Read the model definition and answer for the solid it produces. Units are mm, in the model's axes. A direction names the side the tool comes from. Round coordinates to 2 decimals unless told otherwise and drop trailing zeros. Write each loop counter-clockwise with the first axis right and the second up, starting at its lowest first coordinate (ties: lowest second). Pieces come first, ordered by that corner, then holes. Notation, with made-up numbers: (83.25, -30.5) - (117.25, -30.5) arc R5 ccw to (117.25, -22.5) - close; hole circle Ø6 at (31, 60.5). An arc over 180 degrees is marked (long way). One line per item, written item: value. Start each with the question number.
(1) A cutting plane is placed at C-C, the plane y = 11. Determine the outline of the cut face in (x, z).
(2) A cutting plane is placed at B-B, the plane y = 14. Determine the outline of the cut face in (x, z).
(3) For faces 4 (the face through (7.645, 12.352, 1.479)), 5 (the face through (-2.6, 9.3, 3)), determine the directions among +Z, -Z, +X, -X, +Y, -Y from which every point of the face is accessible in a straight line to the end or side of a thin tool.
(4) Find the intervals of material crossed by L1, parallel to Y at x = -8.25, z = 2.3; L2, parallel to X at y = 0, z = 0.8; L3, parallel to X at y = 3, z = 1, in increasing order.
(5) Flat-ended cylindrical pins translate along their axes: pin 1 Ø1.5 at (x, z) = (-0.5, 1.5) entering from +Y; pin 2 Ø6 at (x, y) = (-5, -3) entering from -Z. Find the tip coordinate at first contact, or state that the pin passes through.
(6) A cutting plane is placed at A-A, the plane x = 0. Determine the outline of the cut face in (y, z), plus the area to 3 significant figures.
(7) The mould has two halves that part along Y. Classify faces 1 (the face through (-0.38, -11.494, 1.479)), 2 (the face through (-2.6, 9.3, 0)), 3 (the face through (0.1, 11.5, 1.5)): +Y half, -Y half, draft (parallel to the pull), parting line (faces both ways), or undercut.
from build123d import *

# Parameters (mm, degrees)
CYLINDER003_R     = 4
CYLINDER003_DEPTH = 3
CYLINDER002_R     = 4
CYLINDER002_DEPTH = 3
CYLINDER001_R     = 9.5
CYLINDER001_DEPTH = 10
CYLINDER_R        = 11.5
CYLINDER_DEPTH    = 3
FILLET_R          = 0.3


with BuildPart() as cilindro003:
    # Cylinder003 → Cylinder003 (new body)
    with BuildSketch(Plane(origin=(3, 2, 0), x_dir=(1, 0, 0), z_dir=(0, 0, 1))):
        Circle(CYLINDER003_R)
    extrude(amount=CYLINDER003_DEPTH)


with BuildPart() as cilindro002:
    # Cylinder002 → Cylinder002 (new body)
    with BuildSketch(Plane.XY):
        Circle(CYLINDER002_R)
    extrude(amount=CYLINDER002_DEPTH)


with BuildPart() as cut001:
    # Cut001 base: copy of Cilindro002
    add(cilindro002.part)

    # Cut001: cut Cilindro003
    add(cilindro003.part, mode=Mode.SUBTRACT)


with BuildPart() as cut001_1:
    # Cut001 placement: moved
    add(cut001.part.moved(Location((-7, 11, 0))))


with BuildPart() as obj1:
    # Part__Mirroring: instance of Cut001
    add(cut001_1.part.mirror(Plane(origin=(0, 0, 0), x_dir=(0, -1, 0), z_dir=(1, 0, 0))))


with BuildPart() as obj1_1:
    # Part__Mirroring placement: moved
    add(obj1.part.moved(Location((0, 1, 0))))


with BuildPart() as cilindro_interior:
    # Cylinder001 → Cylinder001 (new body)
    with BuildSketch(Plane.XY.offset(-3)):
        Circle(CYLINDER001_R)
    extrude(amount=CYLINDER001_DEPTH)


with BuildPart() as obj2:
    # Cylinder → Cylinder (new body)
    with BuildSketch(Plane.XY):
        Circle(CYLINDER_R)
    extrude(amount=CYLINDER_DEPTH)

    # Cut: cut cilindro-interior
    add(cilindro_interior.part, mode=Mode.SUBTRACT)


with BuildPart() as obj3:
    # Cut002 base: copy of Cilindro002
    add(cilindro002.part)

    # Cut002: cut Cilindro003
    add(cilindro003.part, mode=Mode.SUBTRACT)


with BuildPart() as obj3_1:
    # Cut002 placement: moved
    add(obj3.part.moved(Location((-7, 12, 0))))

    # Fusion: union obj1, obj2
    add(obj1_1.part)
    add(obj2.part)

    # Fillet
    fillet_edges = [obj3_1.edges().sort_by_distance(p)[0] for p in [
        (-7.480676, 15.971014, 1.5),
        (7.480676, 15.971014, 1.5),
    ]]
    fillet(fillet_edges, radius=FILLET_R)


solid = obj3_1.part
Here are the results:
1. outline: (-10.87, 0) - (-6.65, 0) - (-6.65, 3) - (-10.87, 3) - close; (-3.35, 0) - (3.35, 0) - (3.35, 3) - (-3.35, 3) - close; (6.65, 0) - (10.87, 0) - (10.87, 3) - (6.65, 3) - close
2. outline: (-10.46, 0) - (-8, 0) - (-8, 3) - (-10.46, 3) - close; (8, 0) - (10.46, 0) - (10.46, 3) - (8, 3) - close
3. face 4: +Z, -Z
3. face 5: +Z, +X, -X, +Y, -Y
4. L1: -8.01 to -4.71, 4.71 to 8.01, 8.2 to 15.8
4. L2: -11.5 to -9.5, 9.5 to 11.5
4. L3: -11.1 to -9.01, 9.01 to 11.1
5. pin 1: y = 11.5
5. pin 2: through
6. outline: (-11.5, 0) - (-9.5, 0) - (-9.5, 3) - (-11.5, 3) - close; (9.5, 0) - (11.5, 0) - (11.5, 3) - (9.5, 3) - close
6. area: 12.0 mm²
7. face 1: undercut
7. face 2: draft
7. face 3: +Y half
